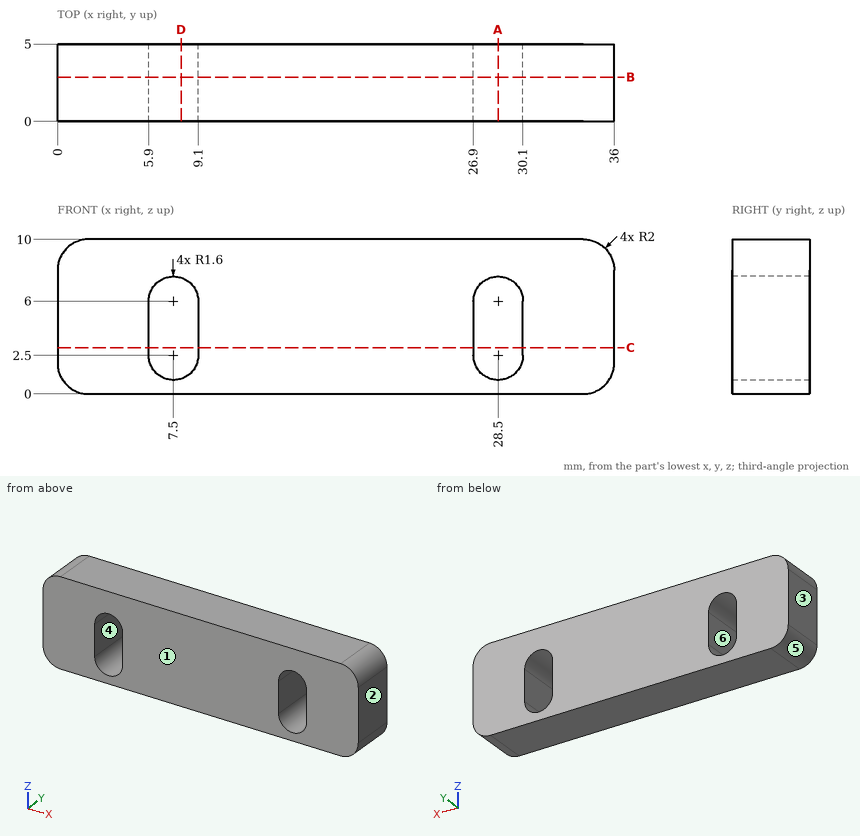
Verification items for this drawing (mm, ordinates from the low corner). A direction names the side the tool comes from. Give positions to 0.01 mm unless a question says otherwise; leave off trailing zeros. Write each loop counter-clockwise with the first axis right and the second up, starting at its lowest first coordinate (ties: lowest second). Pieces come first, ordered by that corner, then holes. Notation, with made-up numbers: (-39.75, -33) -> (-35.75, -33) arc R28 ccw to (-35.75, -3) -> close; hole circle Ø6 at (71, -19.5). An arc over 180 degrees is marked (long way). Use CSV: the item, a comma, the result in double quotes. Start each with the question number.
Q1. Cross-section at A-A on x = 28.5. Enter the section's corners in (y, z).
Q2. Release check for a two-part mould opening along X. For the marked faces 1, 2, 3 and 4 record: +X half, -X half, draft (parallel to the pull), parting line (faces both ways), or undercut.
Q3. Tool access check on the marked faces 5 and 6. Record the directions out of +Z, -Z, +X, -X, +Y, -Y that give a thin tool (end or side, any length) a straight path to the whole face; none if there is none.
Q4. Scan lines: line 1 along X through (y, z) = (0.9, 5.25); line 2 along X through (y, z) = (3.2, 7.25); line 3 along Z through (x, y) = (8, 3.75). Record each from-to range of solid material in increasing order.
Q5. Cross-section at B-B on y = 2.85. Enter the section's corners in (x, z).
Q6. Cross-section at D-D on x = 8. Enter the section's corners in (y, z).
Q7. Cross-section at C-C on z = 3. Enter the section's corners in (x, y).
Working result:
1,outline,"(0, 0) -> (5, 0) -> (5, 0.9) -> (0, 0.9) -> close; (0, 7.6) -> (5, 7.6) -> (5, 10) -> (0, 10) -> close"
2,face 1,"draft"
2,face 2,"+X half"
2,face 3,"-X half"
2,face 4,"undercut"
3,face 5,"-Z, -X, +Y, -Y"
3,face 6,"+Y, -Y"
4,line 1,"x = 0 to 5.9, 9.1 to 26.9, 30.1 to 36"
4,line 2,"x = 0 to 6.5, 8.5 to 27.5, 29.5 to 36"
4,line 3,"z = 0 to 0.98, 7.52 to 10"
5,outline,"(0, 2) arc R2 ccw to (2, 0) -> (34, 0) arc R2 ccw to (36, 2) -> (36, 8) arc R2 ccw to (34, 10) -> (2, 10) arc R2 ccw to (0, 8) -> close; hole (5.9, 2.5) arc R1.6 ccw to (9.1, 2.5) -> (9.1, 6) arc R1.6 ccw to (5.9, 6) -> close; hole (26.9, 2.5) arc R1.6 ccw to (30.1, 2.5) -> (30.1, 6) arc R1.6 ccw to (26.9, 6) -> close"
6,outline,"(0, 0) -> (5, 0) -> (5, 0.98) -> (0, 0.98) -> close; (0, 7.52) -> (5, 7.52) -> (5, 10) -> (0, 10) -> close"
7,outline,"(0, 0) -> (5.9, 0) -> (5.9, 5) -> (0, 5) -> close; (9.1, 0) -> (26.9, 0) -> (26.9, 5) -> (9.1, 5) -> close; (30.1, 0) -> (36, 0) -> (36, 5) -> (30.1, 5) -> close"
